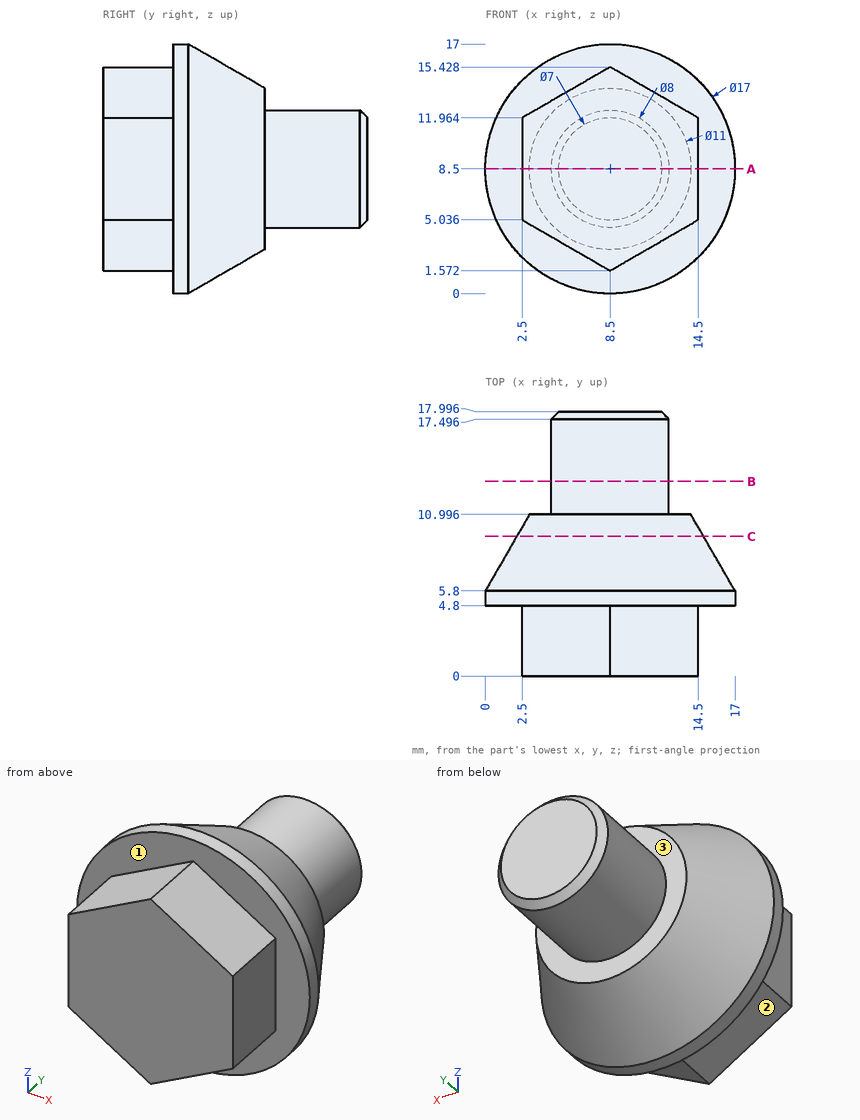
Could you check a few things on this drawing? It's one solid part, dimensions in mm from its lowest x, y, z. A direction names the side the tool comes from. Give positions to 0.01 mm unless a question says otherwise; leave off trailing zeros. Order: outer loops, then holes, each group sorted by start corner. A loop starts at its lowest first (then second) coordinate and runs counter-clockwise, first axis right, second up. Notation, with made-up numbers: (-39, 75.5) - (13, 75.5) arc R17 ccw to (13, 108.5) - close; hole circle Ø4 at (81, 81). An arc over 180 degrees is marked (long way). Return JSON: item names as keys, results as strings. Group by question number.
Q1. Suppose I cut it at B-B, the plane y = 13.25. Please give me the cut outline in (x, z), and give its area (3 significant figures).
Q2. Will these pins go through, and if not, where does the flat tip stop? pin 1 Ø6 at (y, z) = (16, 11.5) entering from +X; pin 2 Ø2.5 at (y, z) = (1, 7) entering from +X; pin 3 Ø1.5 at (x, y) = (7, 10) entering from +Z.
Q3. Suppose I cut it at C-C, the plane y = 9.5. Please give me the cut outline in (x, z), and give its area (3 significant figures).
Q4. Which directions (+Z, -Z, +X, -X, +Y, -Y) give clear straight access to the entire face, cutting with the end or side of a thin tool? Please do the marked faces 1, 2 and 3.
Q5. Please list where these lines run through material, in increasing order: line 1 along X through (y, z) = (4.75, 8.5); line 2 along Y through (x, z) = (10, 12.5); line 3 along Z through (x, y) = (10, 4). Write a range as [from, to].
Q6. Suppose I cut it at A-A, the plane z = 8.5. Please give me the cut outline in (x, y).
Resolved:
{
 "1": {"outline": "circle Ø8 at (8.5, 8.5)", "area": "50.3 mm2"},
 "2": {"pin 1": "stops at x = 12.5", "pin 2": "stops at x = 14.5", "pin 3": "stops at z = 14.86"},
 "3": {"outline": "circle Ø12.73 at (8.5, 8.5)", "area": "127 mm2"},
 "4": {"face 1": "-Y", "face 2": "-Z, -X, -Y", "face 3": "+Y"},
 "5": {"line 1": "x = [2.5, 14.5]", "line 2": "y = [0, 11]", "line 3": "z = [2.44, 14.56]"},
 "6": {"outline": "(0, 4.8) - (2.5, 4.8) - (2.5, 0) - (14.5, 0) - (14.5, 4.8) - (17, 4.8) - (17, 5.8) - (14, 11) - (12.5, 11) - (12.5, 17.5) - (12, 18) - (5, 18) - (4.5, 17.5) - (4.5, 11) - (3, 11) - (0, 5.8) - close"}
}
